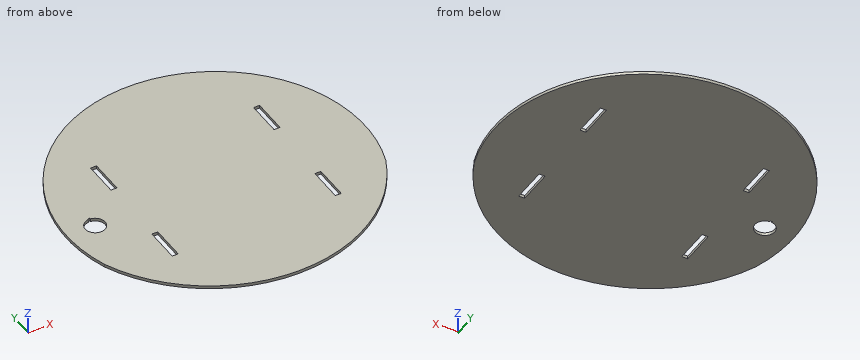
```python
from build123d import *

# Parameters (mm, degrees)
ESBO_O1_W                = 6
ESBO_O1_H                = 35
RESSALTO_EXTRUS_O1_DEPTH = 3


with BuildPart() as part:
    # Esboço1 → Ressalto-extrusão1 (new body)
    with BuildSketch(Plane.XY):
        with BuildLine():
            ThreePointArc((141.421356237, -50), (0, 150), (-141.421356237, -50))
            ThreePointArc((-141.421356237, -50), (0, -142.957457878), (141.421356237, -50))
        make_face()
        with BuildLine():
            Line((-120.321356237, 11), (-122.521356237, 11))
            Line((-122.521356237, 11), (-122.521356237, 9.939315872))
            ThreePointArc((-122.521356237, 9.939315872), (-121.421356237, -10), (-120.321356237, 9.939315872))
            Line((-120.321356237, 9.939315872), (-120.321356237, 11))
        make_face(mode=Mode.SUBTRACT)
        with Locations((-82, -52.5)):
            Rectangle(ESBO_O1_W, ESBO_O1_H, mode=Mode.SUBTRACT)
        with Locations((-82, 52.5)):
            Rectangle(ESBO_O1_W, ESBO_O1_H, mode=Mode.SUBTRACT)
        with Locations((82, -52.5)):
            Rectangle(ESBO_O1_W, ESBO_O1_H, mode=Mode.SUBTRACT)
        with Locations((82, 52.5)):
            Rectangle(ESBO_O1_W, ESBO_O1_H, mode=Mode.SUBTRACT)
    extrude(amount=RESSALTO_EXTRUS_O1_DEPTH)


solid = part.part
```
Geometry check sheet. Reference: the model listing, model coordinates, mm. Coordinates: 2 decimals unless noted, no trailing zeros. Order: outer loops, then holes, each group sorted by start corner. A loop starts at its lowest first (then second) coordinate and runs counter-clockwise, first axis right, second up. Notation, with made-up numbers: (78, 73) - (86, 73) arc R19 cw to (86, 101) - close; hole circle Ø7 at (57.5, 57). An arc over 180 degrees is marked (long way). Answer as a JSON object with one key per item and string values. Group by question number.
Item 1: Sectioned sample at D-D, the plane x = 123. Record the cut outline in (y, z), and give its area (3 significant figures).
Item 2: Depth check by flat-ended pin: pin 1 Ø1.5 at (y, z) = (-28.5, 0.5) entering from -X; pin 2 Ø1 at (x, z) = (-6, 1.5) entering from -Y; pin 3 Ø0.9 at (y, z) = (-48.5, 1.5) entering from -X. Enter the tip coordinate at first touch or a pass-through.
Item 3: Sectioned sample at B-B, the plane z = 1.1. Record the cut outline in (x, y), and give its area (3 significant figures).
Item 4: Sectioned sample at A-A, the plane y = 0. Record the cut outline in (x, z), and give its area (3 significant figures).
Item 5: Sectioned sample at C-C, the plane y = -46. Record the cut outline in (x, z), and give its area (3 significant figures).
Item 6: Scan lines: probe 1 along X at (y, z) = (0, 1.2); probe 2 along X at (y, z) = (45, 1.55); probe 3 along X at (y, z) = (53, 0.8). Record each from-to range of solid material in increasing order.
Resolved:
{
 "1": {"outline": "(-81.66, 0) - (85.85, 0) - (85.85, 3) - (-81.66, 3) - close", "area": "503 mm^2"},
 "2": {"pin 1": "x = -147.41", "pin 2": "y = -142.86", "pin 3": "x = -142.1"},
 "3": {"outline": "(-141.42, -50) arc R154.05 ccw to (141.42, -50) arc R150 ccw (long way) to start; hole (-122.52, 9.94) arc R10 ccw (long way) to (-120.32, 9.94) - (-120.32, 11) - (-122.52, 11) - close; hole (-85, -70) - (-79, -70) - (-79, -35) - (-85, -35) - close; hole (-85, 35) - (-79, 35) - (-79, 70) - (-85, 70) - close; hole (79, -70) - (85, -70) - (85, -35) - (79, -35) - close; hole (79, 35) - (85, 35) - (85, 70) - (79, 70) - close", "area": "67,900 mm^2"},
 "4": {"outline": "(-150, 0) - (-131.42, 0) - (-131.42, 3) - (-150, 3) - close; (-111.42, 0) - (150, 0) - (150, 3) - (-111.42, 3) - close", "area": "840 mm^2"},
 "5": {"outline": "(-142.77, 0) - (-85, 0) - (-85, 3) - (-142.77, 3) - close; (-79, 0) - (79, 0) - (79, 3) - (-79, 3) - close; (85, 0) - (142.77, 0) - (142.77, 3) - (85, 3) - close", "area": "821 mm^2"},
 "6": {"probe 1": "-150 to -131.42, -111.42 to 150", "probe 2": "-143.09 to -85, -79 to 79, 85 to 143.09", "probe 3": "-140.32 to -85, -79 to 79, 85 to 140.32"}
}
